from build123d import *

# Parameters (mm, degrees)
SKETCH_W    = 40
SKETCH_H    = 30
SKETCH_W_2  = 34
SKETCH_H_2  = 24
PAD_DEPTH   = 4
FILLET_R    = 3
FILLET001_R = 1


with BuildPart() as part:
    # Sketch → Pad (new body)
    with BuildSketch(Plane.XY):
        Rectangle(SKETCH_W, SKETCH_H)
        Rectangle(SKETCH_W_2, SKETCH_H_2, mode=Mode.SUBTRACT)
    extrude(amount=PAD_DEPTH)

    # Fillet
    fillet_edges = [part.edges().sort_by_distance(p)[0] for p in [
        (-20, -15, 2),
        (20, -15, 2),
        (20, 15, 2),
        (-20, 15, 2),
    ]]
    fillet(fillet_edges, radius=FILLET_R)

    # Fillet001
    fillet001_edges = [part.edges().sort_by_distance(p)[0] for p in [
        (17, 12, 2),
        (-17, 12, 2),
        (-17, -12, 2),
        (17, -12, 2),
    ]]
    fillet(fillet001_edges, radius=FILLET001_R)


solid = part.part
Input: part model. Units: mm. Frame: model coordinates. A direction names the side the tool comes from. Coordinates: 2 decimals unless noted, no trailing zeros. Loops run counter-clockwise (first coordinate to the right, second up) from the corner with the lowest first, then second, coordinate; pieces in that order, holes last.
(1) First-contact query: pin 1 Ø10 at (x, y) = (-6.5, -11.5) entering from -Z. Flat tip, straight axial feed; report the tip coordinate or a pass-through.
(2) Section A-A on y = 5.75. Return the cut outline in (x, z).
(3) Section B-B on z = 2.2. Return the cut outline in (x, y), then the cut area to 3 significant figures.
(4) Set-up query: faces 4 (the face through (19.1, 14.14, 2.03)), 5 (the face through (16.699, -11.715, 2.028)). Return all of +Z, -Z, +X, -X, +Y, -Y with unobstructed straight access to the full face (end or side cutting, diameter ignored); none if empty.
(5) Material intervals for probe 1 along X at (y, z) = (-10, 1.5); probe 2 along Y at (x, z) = (-11.5, 1.85); probe 3 along X at (y, z) = (-11.5, 1.05), sorted ascending.
(6) Section C-C on x = -3. Return the cut outline in (y, z), then the cut area to 3 significant figures.
(7) Pull-direction query (X, two-part tool) for faces 1 (the face through (-16.699, 11.715, 2.028)), 2 (the face through (0, -15, 2)), 3 (the face through (-20, 0, 2)); classes: released by +X, released by -X, zero draft, split by the parting line, or undercut.
Data:
1. pin 1: stops at z = 0
2. outline: (-20, 0) - (-17, 0) - (-17, 4) - (-20, 4) - close; (17, 0) - (20, 0) - (20, 4) - (17, 4) - close
3. outline: (-20, -12) arc R3 ccw to (-17, -15) - (17, -15) arc R3 ccw to (20, -12) - (20, 12) arc R3 ccw to (17, 15) - (-17, 15) arc R3 ccw to (-20, 12) - close; hole (-17, -11) arc R1 ccw to (-16, -12) - (16, -12) arc R1 ccw to (17, -11) - (17, 11) arc R1 ccw to (16, 12) - (-16, 12) arc R1 ccw to (-17, 11) - close
3. area: 377 mm2
4. face 4: +Z, -Z, +X, +Y
4. face 5: +Z, -Z
5. probe 1: x = -20 to -17, 17 to 20
5. probe 2: y = -15 to -12, 12 to 15
5. probe 3: x = -20 to -16.87, 16.87 to 20
6. outline: (-15, 0) - (-12, 0) - (-12, 4) - (-15, 4) - close; (12, 0) - (15, 0) - (15, 4) - (12, 4) - close
6. area: 24.0 mm2
7. face 1: undercut
7. face 2: zero draft
7. face 3: released by -X
